```python
from build123d import *

# Parameters (mm, degrees)
SKETCH_1_R          = 12.5
EXTRUDE_1_DEPTH     = 19
SKETCH_2_R          = 3.5
EXTRUDE_2_DEPTH     = 2.5
SKETCH_3_R          = 2
EXTRUDE_3_DEPTH     = 22.5
SKETCH_4_W          = 6.562487183
SKETCH_4_H          = 1.182107807
CUT_EXTRUDE_1_DEPTH = 13
SKETCH_5_R          = 12.2
EXTRUDE_5_DEPTH     = 32.5
SKETCH_6_R          = 3.5
EXTRUDE_6_DEPTH     = 3
SKETCH_7_R          = 1
EXTRUDE_7_DEPTH     = 5
SKETCH_8_R          = 1.25
CUT_EXTRUDE_2_DEPTH = 5
SKETCH_9_W          = 0.5
SKETCH_9_H          = 4
EXTRUDE_8_DEPTH     = 5.5


with BuildPart() as part:
    # 스케치1 → 보스-돌출1 (new body)
    with BuildSketch(Plane.XY):
        Circle(SKETCH_1_R)
    extrude(amount=EXTRUDE_1_DEPTH)

    # 스케치2 → 보스-돌출2 (add)
    with BuildSketch(Plane.XY.offset(19)):
        Circle(SKETCH_2_R)
    extrude(amount=EXTRUDE_2_DEPTH)

    # 스케치3 → 보스-돌출3 (add)
    with BuildSketch(Plane.XY.offset(21.5)):
        Circle(SKETCH_3_R)
    extrude(amount=EXTRUDE_3_DEPTH)

    # 스케치4 → 컷-돌출1 (cut)
    with BuildSketch(Plane.XY.offset(44)):
        with Locations((0.048491285, 1.591053903)):
            Rectangle(SKETCH_4_W, SKETCH_4_H)
    extrude(amount=-CUT_EXTRUDE_1_DEPTH, mode=Mode.SUBTRACT)

    # 스케치5 → 보스-돌출5 (add)
    with BuildSketch(Plane(origin=(0, 0, 0), x_dir=(-1, 0, 0), z_dir=(0, 0, -1))):
        Circle(SKETCH_5_R)
    extrude(amount=EXTRUDE_5_DEPTH)

    # 스케치6 → 보스-돌출6 (add)
    with BuildSketch(Plane(origin=(0, 0, -32.5), x_dir=(-1, 0, 0), z_dir=(0, 0, -1))):
        Circle(SKETCH_6_R)
    extrude(amount=EXTRUDE_6_DEPTH)

    # 스케치7 → 보스-돌출7 (add)
    with BuildSketch(Plane(origin=(0, 0, -35.5), x_dir=(-1, 0, 0), z_dir=(0, 0, -1))):
        Circle(SKETCH_7_R)
    extrude(amount=EXTRUDE_7_DEPTH)

    # 스케치8 → 컷-돌출2 (cut)
    with BuildSketch(Plane.XY.offset(19)):
        with Locations((0, 8.5)):
            Circle(SKETCH_8_R)
        with Locations((0, -8.5)):
            Circle(SKETCH_8_R)
    extrude(amount=-CUT_EXTRUDE_2_DEPTH, mode=Mode.SUBTRACT)

    # 스케치9 → 보스-돌출8 (add)
    with BuildSketch(Plane(origin=(0, 0, -32.5), x_dir=(-1, 0, 0), z_dir=(0, 0, -1))):
        with Locations((-9.25, 0)):
            Rectangle(SKETCH_9_W, SKETCH_9_H)
        with Locations((9.25, 0)):
            Rectangle(SKETCH_9_W, SKETCH_9_H)
    extrude(amount=EXTRUDE_8_DEPTH)


solid = part.part
```
The model under review builds one solid part; all positions refer to its coordinate system, in mm. A direction names the side the tool comes from. Round coordinates to 2 decimals unless told otherwise and drop trailing zeros. Order: outer loops, then holes, each group sorted by start corner. A loop starts at its lowest first (then second) coordinate and runs counter-clockwise, first axis right, second up.
Item 1: Add section D-D, the plane y = -8.5. State the section outline as (x, z) points.
Working result:
outline: (-9.17, 0) - (-8.75, 0) - (-8.75, -32.5) - (8.75, -32.5) - (8.75, 0) - (9.17, 0) - (9.17, 19) - (1.25, 19) - (1.25, 14) - (-1.25, 14) - (-1.25, 19) - (-9.17, 19) - close
Item 2: To check wall thickness, follow probe 1 along Y at (x, z) = (0, 15); probe 2 along Z at (x, y) = (2.5, 1.5); probe 3 along X at (y, z) = (-0.5, -22). State the ranges of each line that lie inside material, in increasing order.
Working result:
probe 1: y = -12.5 to -9.75, -7.25 to 7.25, 9.75 to 12.5
probe 2: z = -35.5 to 21.5
probe 3: x = -12.19 to 12.19
Item 3: For pin 1 (2 mm diameter, centred on x = 2, z = 29.5, fed in from +Y); pin 2 (8 mm diameter, centred on x = -1.5, z = -8, fed in from -Y); pin 3 (4 mm diameter, centred on x = 0.5, z = 39.5, fed in from +Y); pin 4 (1.5 mm diameter, centred on y = 3, z = 31.5, fed in from -X), all flat-tipped, find the tip position at first contact; note any pin that passes through.
Working result:
pin 1: stops at y = 1.73
pin 2: stops at y = -12.2
pin 3: stops at y = 1
pin 4: passes through
Item 4: Draft analysis for pull direction X (two halves, no side actions). For faces 1 (the flat face through (-9, 0, -35)), 2 (the cylindrical face through (3.233, -1.341, 20.232)), 3 (the flat face through (9.5, 0, -35)), state which applies: released by +X, released by -X, zero draft, split by the parting line, or undercut.
Working result:
face 1: undercut
face 2: split by the parting line
face 3: released by +X
Item 5: Machinability: for faces 4 (the cylindrical face through (-3.233, -1.341, -33.979)), 5 (the flat face through (-9.5, 0, -35)), 6 (the flat face through (0, 1, 38)), 7 (the flat face through (0, 0, -40.5)), 8 (the flat face through (3, -3, 19)), which of the approach directions +Z, -Z, +X, -X, +Y, -Y give a long, thin tool a straight path to every point of the face, cutting with its end or side? Answer none if there is none.
Working result:
face 4: -Z
face 5: -Z, -X, +Y, -Y
face 6: +Z, +X, -X, +Y
face 7: -Z, +X, -X, +Y, -Y
face 8: +Z
Item 6: Add section C-C, the plane z = 8. State the section outline as (x, y) points, and give its area (3 significant figures).
Working result:
outline: circle Ø25 at (0, 0)
area: 491 mm2
